Model file for the job. Use its own axes, mm. A direction names the side the tool comes from. Round coordinates to 2 decimals unless told otherwise and drop trailing zeros. Write each loop counter-clockwise with the first axis right and the second up, starting at its lowest first coordinate (ties: lowest second). Pieces come first, ordered by that corner, then holes.
Autodesk Inventor part; units mm, degrees
ref_plane "YZ Plane" through (0, 0, 0) normal (1, 0, 0) x (0, 1, 0)
ref_plane "XZ Plane" through (0, 0, 0) normal (0, 1, 0) x (-1, 0, 0)
ref_plane "XY Plane" through (0, 0, 0) normal (0, 0, 1) x (1, 0, 0)
sketch "Sketch1" plane through (0, 0, 0) normal (0, 1, 0) x (-1, 0, 0)
  circle A0 centre (0, 0) radius 4.45
  circle A1 centre (0, 0) radius 2.55
  dimension "d0" = 8.9
  dimension "d1" = 5.1
extrude "Extrusion1" add sketch "Sketch1" along normal blind 18
sketch "Sketch2" plane through (0, 18, 0) normal (0, 1, 0) x (1, 0, 0)
  line L0 (25, -25) -> (-25, -25)
  line L1 (-25, -25) -> (-25, 25)
  line L2 (-25, 25) -> (25, 25)
  line L3 (25, 25) -> (25, -25)
  line L4 (25, -25) -> (-25, 25) construction
  line L5 (-25, -25) -> (25, 25) construction
  line L6 (7.5, -12.875) -> (-7.5, -12.875)
  line L7 (-7.5, -12.875) -> (-7.5, 12.875)
  line L8 (-7.5, 12.875) -> (7.5, 12.875)
  line L9 (7.5, 12.875) -> (7.5, -12.875)
  line L10 (7.5, -12.875) -> (-7.5, 12.875) construction
  line L11 (-7.5, -12.875) -> (7.5, 12.875) construction
  line L12 (-7.5, 12.875) -> (-7.5, 17.125)
  circle A0 centre (-7.5, 15) radius 2.125
  circle A1 centre (7.5, 15) radius 2.125
  line L13 (-7.5, -12.875) -> (-7.5, -17.125)
  circle A2 centre (-7.5, -15) radius 2.125
  circle A3 centre (7.5, -15) radius 2.125
  circle A4 centre (0, 0) radius 4.45
  circle A5 centre (0, 0) radius 22.5
  dimension "d7" = 50
  dimension "d8" = 50
  dimension "d9" = 15
  dimension "d10" = 25.75
  dimension "d11" = 4.25
  dimension "d12" = 4.25
  dimension "d13" = 45
extrude "Extrusion2" add sketch "Sketch2" along normal blind 5 contours L6 L7 L8 L9 | A4 | A5
fillet "Fillet1" radius 2 2 edges at (-22.5, 18, 0) (-22.5, 23, 0)
properties part number "mountingnema" material "Aluminum 6061"
1) Cut at C-C on z = 15. Give the number of separate pieces and of enclosed holes in the cut face, and give its area (3 significant figures).
2) Cut at A-A on z = 0. List the corners of the cut face in (x, y), and give its area (3 significant figures).
3) Flat gauge pins, fed straight in: pin 1 Ø3 at (y, z) = (18, 4) entering from -X; pin 2 Ø6.5 at (x, z) = (0, 0) entering from -Y; pin 3 Ø7 at (x, z) = (7.5, -15) entering from -Y; pin 4 Ø5 at (x, y) = (3.5, 4.5) entering from +Z. Where does each tip first touch, or does it go through?
4) Pull direction Z, two halves, no side cores. Call faces 3 (the face through (10.382, 20.493, -19.961)), 4 (the face through (-5, 18, 0)), 5 (the face through (-6.519, 20.465, 13.115)): released by +Z, released by -Z, zero draft, split by the parting line, or undercut.
5) Cut at B-B on y = 12.25. List the corners of the cut face in (x, z).
6) Which spindle directions (+Z, -Z, +X, -X, +Y, -Y) get a long thin tool onto all of the face, cutting with end or side? Do faces 1 (the face through (0, 23, 0)), 2 (the face through (0, 18, 0)). Say none if no direction does.
7) Wall check: probe 1 along Z at (x, y) = (7.5, 20.3) (3 decimals); probe 2 along X at (y, z) = (21.9, -15) (3 decimals); probe 3 along Z at (x, y) = (0, 4.75). Give the ranges that are in metal, low to high.
Result sheet:
1. separate pieces: 3
1. enclosed holes: 0
1. area: 121 mm2
2. outline: (-22.5, 20) arc R2 ccw to (-20.5, 18) - (-4.45, 18) - (-4.45, 0) - (-2.55, 0) - (-2.55, 18) - (2.55, 18) - (2.55, 0) - (4.45, 0) - (4.45, 18) - (20.5, 18) arc R2 ccw to (22.5, 20) - (22.5, 21) arc R2 ccw to (20.5, 23) - (-20.5, 23) arc R2 ccw to (-22.5, 21) - close
2. area: 290 mm2
3. pin 1: stops at x = -22.14
3. pin 2: stops at y = 0
3. pin 3: stops at y = 18
3. pin 4: stops at z = 4.34
4. face 3: split by the parting line
4. face 4: zero draft
4. face 5: undercut
5. outline: circle Ø8.9 at (0, 0); hole circle Ø5.1 at (0, 0)
6. face 1: +Z, -Z, +X, -X, +Y
6. face 2: -Y
7. probe 1: z = -21.213 to -17.125, -12.875 to 12.875, 17.125 to 21.213
7. probe 2: x = -16.482 to -9.625, -5.375 to 5.375, 9.625 to 16.482
7. probe 3: z = -4.45 to -2.55, 2.55 to 4.45
